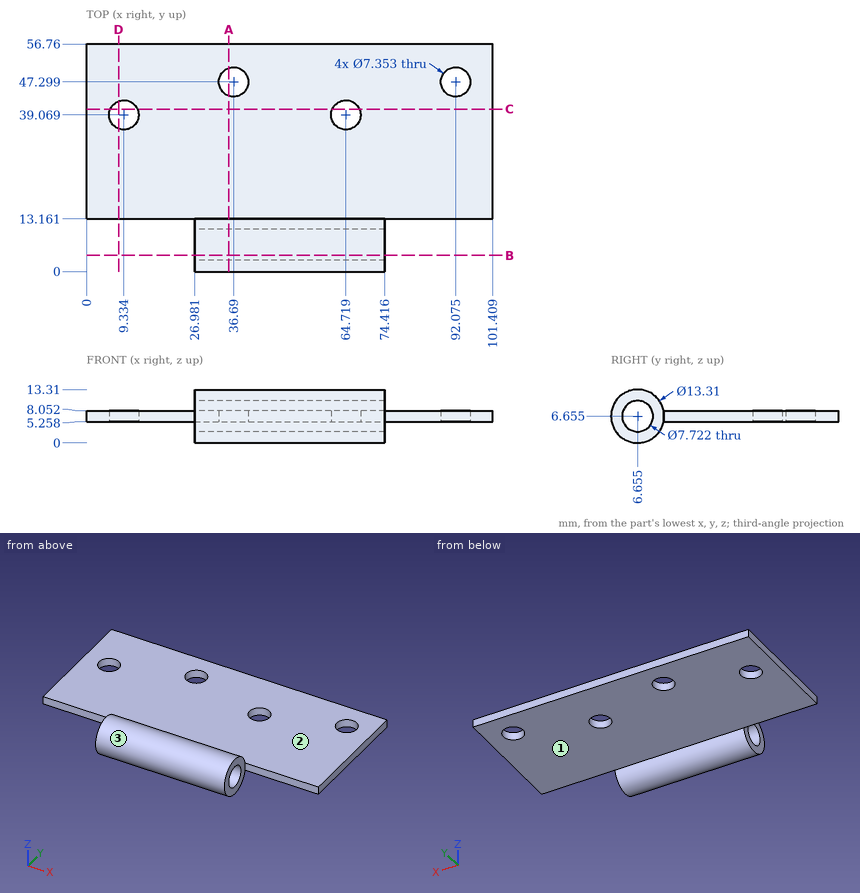
Verification items for this drawing (mm, ordinates from the low corner). A direction names the side the tool comes from. Coordinates: 2 decimals unless noted, no trailing zeros. Order: outer loops, then holes, each group sorted by start corner. A loop starts at its lowest first (then second) coordinate and runs counter-clockwise, first axis right, second up. Notation, with made-up numbers: (70, 37.5) - (117, 37.5) arc R33 ccw to (117, 72.5) - close; hole circle Ø5 at (-32, 32.25). An arc over 180 degrees is marked (long way). Answer in a Markdown table with one row per item. Add a question column.
1. Gauge pin test, flat ends, axial feed: pin 1 Ø3 at (x, z) = (87, 6.5) entering from -Y; pin 2 Ø9.5 at (x, y) = (64.72, 39.07) entering from +Z; pin 3 Ø12 at (x, y) = (73, 42.5) entering from -Z. Record the tip position at first contact, or that the pin passes through.
2. Section check A-A (x = 35.5). Enter the section's corners in (y, z) (1 decimal).
3. Section check C-C (y = 40.5). Enter the section's corners in (x, z).
4. Material ranges on L1, parallel to X at y = 39, z = 5.5 (1 decimal); L2, parallel to Z at x = 73.5, y = 40.5; L3, parallel to X at y = 11, z = 10.25 (1 decimal), recorded low to high. Write a range as [from, to].
5. Access from +Z, -Z, +X, -X, +Y, -Y to the whole of each face (thin tool, end or side, straight path). Record for the marked faces 1, 2 and 3.
6. Section check D-D (x = 8). Enter the section's corners in (y, z) (1 decimal).
7. Section check B-B (y = 4). Enter the section's corners in (x, z) (1 decimal).
Data:
| question | item | result |
|---|---|---|
| 1 | pin 1 | stops at y = 13.16 |
| 1 | pin 2 | stops at z = 8.05 |
| 1 | pin 3 | stops at z = 5.26 |
| 2 | outline | (13.2, 5.3) - (43.8, 5.3) - (43.8, 8.1) - (13.2, 8.1) arc R6.7 ccw (long way) to start; (50.8, 5.3) - (56.8, 5.3) - (56.8, 8.1) - (50.8, 8.1) - close; hole circle Ø7.7 at (6.7, 6.7) |
| 3 | outline | (0, 5.26) - (5.95, 5.26) - (5.95, 8.05) - (0, 8.05) - close; (12.72, 5.26) - (61.33, 5.26) - (61.33, 8.05) - (12.72, 8.05) - close; (68.11, 5.26) - (101.41, 5.26) - (101.41, 8.05) - (68.11, 8.05) - close |
| 4 | L1 | x = [0, 5.7], [13, 61], [68.4, 101.4] |
| 4 | L2 | z = [5.26, 8.05] |
| 4 | L3 | x = [27, 74.4] |
| 5 | face 1 | -Z, +X, -X, +Y |
| 5 | face 2 | +Z, +X, -X, +Y |
| 5 | face 3 | +X, -X |
| 6 | outline | (13.2, 5.3) - (35.6, 5.3) - (35.6, 8.1) - (13.2, 8.1) - close; (42.5, 5.3) - (56.8, 5.3) - (56.8, 8.1) - (42.5, 8.1) - close |
| 7 | outline | (27, 0.6) - (74.4, 0.6) - (74.4, 3.9) - (27, 3.9) - close; (27, 9.5) - (74.4, 9.5) - (74.4, 12.8) - (27, 12.8) - close |
